from build123d import *


# Not quite as in the source:
# - a fillet or chamfer that OpenCascade refuses, or shapes differently, is made with other operations: its cross-section is extruded or revolved along the edge and cut away or added


with BuildPart() as f1:
    # F0 (on Front) → F1 (revolve)
    with BuildSketch(Plane.XZ):
        Polygon((0, 9.525), (0, 0), (347.6625, 0), (347.6625, 9.525), (207.9625, 15.875), (139.7, 15.875), align=None)
    revolve(axis=Axis((173.83125, 0, 0), (1, 0, 0)))

    # F2: fillet of radius 609.6 on 2 edges, made by hand

    # F2_s1 → F2_t2 (revolve, cut)
    with BuildSketch(Plane.XZ):
        with BuildLine():
            ThreePointArc((153.5473965644, 15.875), (139.7035712187, 15.7177852553), (125.8668864684, 15.2462221122))
            Line((125.8668864684, 15.2462221122), (139.7, 15.875))
            Line((139.7, 15.875), (153.5473965644, 15.875))
        make_face()
    revolve(axis=Axis((139.7, 0, 0), (1, 0, 0)), mode=Mode.SUBTRACT)

    # F2_s3 → F2_t4 (revolve, cut)
    with BuildSketch(Plane.XZ):
        with BuildLine():
            ThreePointArc((221.7956135316, 15.2462221122), (207.9589287813, 15.7177852553), (194.1151034356, 15.875))
            Line((194.1151034356, 15.875), (207.9625, 15.875))
            Line((207.9625, 15.875), (221.7956135316, 15.2462221122))
        make_face()
    revolve(axis=Axis((207.9625, 0, 0), (1, 0, 0)), mode=Mode.SUBTRACT)


solid = f1.part
The model under review builds one solid part; all positions refer to its coordinate system, in mm. Round coordinates to 2 decimals unless told otherwise and drop trailing zeros. Loops run counter-clockwise (first coordinate to the right, second up) from the corner with the lowest first, then second, coordinate; pieces in that order, holes last. Notation, with made-up numbers: M 40.5,14 L 72.5,14 A21 cw 72.5,31 Z; hole C 52,-40 d2. An arc over 180 degrees is marked long. Answer as CSV lines item,"result". Start each with the question number.
Item 1: Consider section A-A (x = 185.5). Write out the cut boundary in (y, z) (3 decimals), then the cut area to 3 significant figures.
Item 2: Consider section B-B (x = 259.5). Write out the cut boundary in (y, z), then the cut area to 3 significant figures.
Item 3: Wall thickness on line 1 (Z direction, x = 143, y = -5.5); line 2 (Y direction, x = 152, z = -11); line 3 (Y direction, x = 316.5, z = -10): over which ranges is each line inside the solid? List them lowest first. Write a range as [from, to].
Item 4: Insertion check: P1, Ø2, axis at x = 292, z = -2, coming from the +Y side; P2, Ø3, axis at x = 160.5, z = -7.5, coming from the +Y side; P3, Ø2, axis at x = 115.5, z = 11, coming from the +Y side. Each pin has a flat end and moves straight along its axis. Give the tip position at first contact, or say it passes through.
Answer:
1,outline,"C 0,0 d31.75"
1,area,"792 mm^2"
2,outline,"C 0,0 d27.06"
2,area,"575 mm^2"
3,line 1,"z = [-14.79, 14.79]"
3,line 2,"y = [-11.44, 11.44]"
3,line 3,"y = [-4.44, 4.44]"
4,P1,"stops at y = 12.02"
4,P2,"stops at y = 14.7"
4,P3,"stops at y = 10.88"
